Can you work these out from the model? Positions are in its coordinate system, mm. A direction names the side the tool comes from. Round coordinates to 2 decimals unless told otherwise and drop trailing zeros. Order: outer loops, then holes, each group sorted by start corner. A loop starts at its lowest first (then second) coordinate and runs counter-clockwise, first axis right, second up.
Q1. If I drill on line 1 (Y direction, x = 23.5, z = -4.25); line 2 (Z direction, x = 13, y = -31); line 3 (Z direction, x = 21, y = 8.5), over which ranges is the centre line in solid material (lowest first)?
Q2. If we section it at C-C (x = 14): Please give me the cut outline in (y, z).
Q3. Will these pins go through, and if not, where does the flat tip stop? P1, Ø8, axis at x = -26.5, z = 6.5, coming from the -Y side; P2, Ø5, axis at x = 0, y = -28.125, coming from the +Z side; P3, Ø3, axis at y = -20.5, z = 3, coming from the +X side; P4, Ø3.5, axis at x = 0, y = 14, coming from the +Z side.
Q4. For faces 4 (the face through (0, -30, -1)), 5 (the face through (20.53, 18.4, -5.42)), 6 (the face through (12.4, -1.2, 9.6)), 7 (the face through (-2, -15, 5)), which set-ups out of +Z, -Z, +X, -X, +Y, -Y let a thin tool reach every point of the face, with its end or its side?
Q5. If we section it at B-B (z = -3): Count the separate pieces of the cut face and the enclosed holes in it, plus the area to 3 significant figures.
Q6. We'd pull the mould along Z, two halves only. Please class faces 1 (the face through (1, 16, 5)), 2 (the face through (2.7, -20.6, -5.6)), 3 (the face through (11, -20, 5)): pulls with the +Z half, pulls with the -Z half, needs draft (parallel to the pull), parting line crosses it, or undercut.
Q7. If we section it at A-A (y = 0): Please give me the cut outline in (x, z) (3 decimals).
from build123d import *
from build123d.topology import SkipClean

# Parameters (mm, degrees)
SKETCH1_R                = 40.125
SKETCH1_R_2              = 6
BOSS_EXTRUDE1_DEPTH      = 4
SKETCH1_3_R              = 6
BOSS_EXTRUDE2_DEPTH      = 4.8
SKETCH2_R                = 7
SKETCH2_R_2              = 6
BOSS_EXTRUDE3_DEPTH      = 1
SKETCH3_R                = 22.5
BOSS_EXTRUDE4_DEPTH      = 10
SKETCH3_3_R              = 24.5
SKETCH3_3_R_2            = 22.5
BOSS_EXTRUDE5_DEPTH      = 1
SKETCH4_R                = 2
CUT_EXTRUDE1_DEPTH       = 60.778518299
SKETCH5_R                = 1.5
CUT_EXTRUDE2_DEPTH       = 60.778518299
SKETCH6_R                = 2.25
CUT_EXTRUDE3_DEPTH       = 5
SKETCH7_R                = 2.8
CUT_EXTRUDE4_DEPTH       = 5
CIRPATTERN2_COUNT        = 4
SKETCH8_R                = 1.5
BOSS_EXTRUDE6_DEPTH      = 11
FILLET1_R                = 3
SKETCH8_2_R              = 1.5
CUT_EXTRUDE5_DEPTH       = 59.446824122
CIRPATTERN3_COUNT        = 3
FILLET1_OF_CIRPATTERN3_R = 3
CIRPATTERN1_COUNT        = 6
SKETCH6_2_R              = 2.25
SKETCH6_2_R_2            = 1.5
BOSS_EXTRUDE7_DEPTH      = 5


with BuildPart() as part:
    # Sketch1 → Boss-Extrude1 (new body)
    # profile 1 of 4: a face of its own
    with BuildSketch(Plane.XY):
        Circle(SKETCH1_R)
        with Locations((0, 28.125)):
            Circle(SKETCH1_R_2, mode=Mode.SUBTRACT)
        with Locations((24.356964481, -14.0625)):
            Circle(SKETCH1_R_2, mode=Mode.SUBTRACT)
        with Locations((-24.356964481, -14.0625)):
            Circle(SKETCH1_R_2, mode=Mode.SUBTRACT)
    # profile 2 of 4: a face of its own
    with BuildSketch(Plane.XY):
        with Locations((0, 28.125)):
            Circle(SKETCH1_R_2)
    # profile 3 of 4: a face of its own
    with BuildSketch(Plane.XY):
        with Locations((-24.356964481, -14.0625)):
            Circle(SKETCH1_R_2)
    # profile 4 of 4: a face of its own
    with BuildSketch(Plane.XY):
        with Locations((24.356964481, -14.0625)):
            Circle(SKETCH1_R_2)
    extrude(amount=BOSS_EXTRUDE1_DEPTH)

    # Sketch1<3> → Boss-Extrude2 (add)
    with BuildSketch(Plane.XY):
        with Locations((0, 28.125)):
            Circle(SKETCH1_3_R)
        with Locations((24.356964481, -14.0625)):
            Circle(SKETCH1_3_R)
        with Locations((-24.356964481, -14.0625)):
            Circle(SKETCH1_3_R)
    extrude(amount=-BOSS_EXTRUDE2_DEPTH)

    # Sketch2 → Boss-Extrude3 (add)
    # profile 1 of 3: a face of its own
    with BuildSketch(Plane(origin=(0, 0, 0), x_dir=(-1, 0, 0), z_dir=(0, 0, -1))):
        with Locations(Location((0, 28.125, 0), (0, 0, 180))):
            Circle(SKETCH2_R)
        with Locations(Location((0, 28.125, 0), (0, 0, 180))):
            Circle(SKETCH2_R_2, mode=Mode.SUBTRACT)
    # profile 2 of 3: a face of its own
    with BuildSketch(Plane(origin=(0, 0, 0), x_dir=(-1, 0, 0), z_dir=(0, 0, -1))):
        with Locations(Location((-24.356964481, -14.0625, 0), (0, 0, 180))):
            Circle(SKETCH2_R)
        with Locations(Location((-24.356964481, -14.0625, 0), (0, 0, 180))):
            Circle(SKETCH2_R_2, mode=Mode.SUBTRACT)
    # profile 3 of 3: a face of its own
    with BuildSketch(Plane(origin=(0, 0, 0), x_dir=(-1, 0, 0), z_dir=(0, 0, -1))):
        with Locations(Location((24.356964481, -14.0625, 0), (0, 0, 180))):
            Circle(SKETCH2_R)
        with Locations(Location((24.356964481, -14.0625, 0), (0, 0, 180))):
            Circle(SKETCH2_R_2, mode=Mode.SUBTRACT)
    extrude(amount=BOSS_EXTRUDE3_DEPTH)

    # Sketch3 → Boss-Extrude4 (add)
    with BuildSketch(Plane.XY.offset(4)):
        Circle(SKETCH3_R)
    extrude(amount=BOSS_EXTRUDE4_DEPTH)

    # Sketch3<3> → Boss-Extrude5 (add)
    with BuildSketch(Plane.XY.offset(4)):
        Circle(SKETCH3_3_R)
        Circle(SKETCH3_3_R_2, mode=Mode.SUBTRACT)
    extrude(amount=BOSS_EXTRUDE5_DEPTH)

    # Sketch4 → Cut-Extrude1 (cut, through all)
    with BuildSketch(Plane.XY.offset(14)):
        with Locations((0, 14)):
            Circle(SKETCH4_R)
        with Locations((14, 0)):
            Circle(SKETCH4_R)
        with Locations((0, -14)):
            Circle(SKETCH4_R)
        with Locations((-14, 0)):
            Circle(SKETCH4_R)
    extrude(amount=-CUT_EXTRUDE1_DEPTH, mode=Mode.SUBTRACT)

    # Sketch5 → Cut-Extrude2 (cut, through all)
    with BuildSketch(Plane(origin=(0, 0, -4.8), x_dir=(-1, 0, 0), z_dir=(0, 0, -1))):
        with Locations((0, 28.125)):
            Circle(SKETCH5_R)
        with Locations((24.356964481, -14.0625)):
            Circle(SKETCH5_R)
        with Locations((-24.356964481, -14.0625)):
            Circle(SKETCH5_R)
    extrude(amount=-CUT_EXTRUDE2_DEPTH, mode=Mode.SUBTRACT)

    # Sketch6 → Cut-Extrude3 (cut)
    with BuildSketch(Plane.XY.offset(4)):
        with Locations((0, 28.125)):
            Circle(SKETCH6_R)
    cut_extrude3 = extrude(amount=-CUT_EXTRUDE3_DEPTH, mode=Mode.SUBTRACT)

    # Sketch7 → Cut-Extrude4 (cut)
    with BuildSketch(Plane(origin=(0, 0, 0), x_dir=(-1, 0, 0), z_dir=(0, 0, -1))):
        with Locations((0, 14)):
            Circle(SKETCH7_R)
    cut_extrude4 = extrude(amount=-CUT_EXTRUDE4_DEPTH, mode=Mode.SUBTRACT)

    # CirPattern2: Cut-Extrude4 ×4 about axis
    cirpattern2_axis = Axis((0, 0, 0), (0, 0, 1))
    for i in range(1, CIRPATTERN2_COUNT):
        add(cut_extrude4.rotate(cirpattern2_axis, i * 360 / CIRPATTERN2_COUNT), mode=Mode.SUBTRACT)

    # Sketch8 → Boss-Extrude6 (add)
    with BuildSketch(Plane(origin=(0, 0, 0), x_dir=(-1, 0, 0), z_dir=(0, 0, -1))):
        with BuildLine():
            Line((-26.05133243, 25.026859644), (-15.696526212, 12.595026394))
            ThreePointArc((-15.696526212, 12.595026394), (-17.428761251, 10.0625), (-18.755875925, 7.296077254))
            Line((-18.755875925, 7.296077254), (-34.699562443, 10.047685865))
            ThreePointArc((-34.699562443, 10.047685865), (-31.285167712, 18.0625), (-26.05133243, 25.026859644))
        make_face()
        with Locations((-24.356964481, 14.0625)):
            Circle(SKETCH8_R, mode=Mode.SUBTRACT)
    boss_extrude6 = extrude(amount=BOSS_EXTRUDE6_DEPTH)

    # Fillet1
    fillet1_edges = [part.edges().sort_by_distance(p)[0] for p in [
        (26.05133243, 25.026859644, -5.5),
        (34.699562443, 10.047685865, -5.5),
        (18.755875925, 7.296077254, -5.5),
        (15.696526212, 12.595026394, -5.5),
    ]]
    fillet(fillet1_edges, radius=FILLET1_R)

    # Sketch8<2> → Cut-Extrude5 (cut, through all)
    with SkipClean():  # the faces are left unmerged after this step: merging them gives an invalid solid
        with BuildSketch(Plane(origin=(0, 0, 0), x_dir=(-1, 0, 0), z_dir=(0, 0, -1))):
            with Locations(Location((-24.356964481, 14.0625, 0), (0, 0, 180))):
                Circle(SKETCH8_2_R)
        cut_extrude5 = extrude(amount=-CUT_EXTRUDE5_DEPTH, mode=Mode.SUBTRACT)

    # CirPattern3: Boss-Extrude6, Cut-Extrude5 ×3 about axis
    cirpattern3_axis = Axis((0, 0, 0), (0, 0, 1))
    add([boss_extrude6.rotate(cirpattern3_axis, i * 360 / CIRPATTERN3_COUNT) for i in range(1, CIRPATTERN3_COUNT)])
    add([cut_extrude5.rotate(cirpattern3_axis, i * 360 / CIRPATTERN3_COUNT) for i in range(1, CIRPATTERN3_COUNT)], mode=Mode.SUBTRACT)

    # Fillet1 of CirPattern3
    fillet1_of_cirpattern3_edges = [part.edges().sort_by_distance(p)[0] for p in [
        (-34.699562443, 10.047685865, -5.5),
        (-26.05133243, 25.026859644, -5.5),
        (-15.696526212, 12.595026394, -5.5),
        (-18.755875925, 7.296077254, -5.5),
        (8.648230013, -35.074545509, -5.5),
        (-8.648230013, -35.074545509, -5.5),
        (-3.059349712, -19.891103648, -5.5),
        (3.059349712, -19.891103648, -5.5),
    ]]
    fillet(fillet1_of_cirpattern3_edges, radius=FILLET1_OF_CIRPATTERN3_R)

    # CirPattern1: Cut-Extrude3 ×6 about axis, 2 skipped
    cirpattern1_axis = Axis((0, 0, 0), (0, 0, 1))
    add([cut_extrude3.rotate(cirpattern1_axis, i * 360 / CIRPATTERN1_COUNT) for i in range(1, CIRPATTERN1_COUNT) if i not in (2, 4)], mode=Mode.SUBTRACT)

    # Sketch6<2> → Boss-Extrude7 (add)
    with BuildSketch(Plane.XY.offset(4)):
        with Locations((0, 28.125)):
            Circle(SKETCH6_2_R)
        with Locations(Location((0, 28.125, 0), (0, 0, 180))):
            Circle(SKETCH6_2_R_2, mode=Mode.SUBTRACT)
    extrude(amount=-BOSS_EXTRUDE7_DEPTH)


solid = part.part
Solution:
1. line 1: y = -20 to -15.29, -12.83 to -8.12, 8.11 to 12.83, 15.29 to 21.96
1. line 2: z = 0 to 4
1. line 3: z = -11 to 5
2. outline: (-37.6, 0) - (-2.8, 0) - (-2.8, 5) - (-2, 5) - (-2, 14) - (-17.61, 14) - (-17.61, 5) - (-20.11, 5) - (-20.11, 4) - (-37.6, 4) - close; (2, 5) - (2.8, 5) - (2.8, 0) - (37.6, 0) - (37.6, 4) - (20.11, 4) - (20.11, 5) - (17.61, 5) - (17.61, 14) - (2, 14) - close
3. P1: stops at y = -32.61
3. P2: stops at z = 4
3. P3: stops at x = 35.34
3. P4: passes through
4. face 4: +Z
4. face 5: -Z, +Y
4. face 6: +Z, -Z
4. face 7: -Z
5. separate pieces: 6
5. enclosed holes: 6
5. area: 840 mm2
6. face 1: pulls with the -Z half
6. face 2: needs draft
6. face 3: pulls with the +Z half
7. outline: (-40.125, 0) - (-16.8, 0) - (-16.8, 5) - (-16, 5) - (-16, 14) - (-22.5, 14) - (-22.5, 5) - (-24.5, 5) - (-24.5, 4) - (-40.125, 4) - close; (-12, 5) - (-11.2, 5) - (-11.2, 0) - (11.2, 0) - (11.2, 5) - (12, 5) - (12, 14) - (-12, 14) - close; (16, 5) - (16.8, 5) - (16.8, 0) - (40.125, 0) - (40.125, 4) - (24.5, 4) - (24.5, 5) - (22.5, 5) - (22.5, 14) - (16, 14) - close
